```python
from build123d import *

# Parameters (mm, degrees)
ESBO_O1_W                = 23
ESBO_O1_H                = 23
RESSALTO_EXTRUS_O1_DEPTH = 10.25
CORTE_EXTRUS_O1_REACH    = 21.224
ESBO_O2_R                = 4.2
ESBO_O3_W                = 60
ESBO_O3_H                = 60
RESSALTO_EXTRUS_O2_DEPTH = 7
CORTE_EXTRUS_O2_REACH    = 45.647
ESBO_O4_R                = 1.5
CORTE_EXTRUS_O3_DEPTH    = 2.8
FILETE1_R                = 2
FILETE2_R                = 2


with BuildPart() as part:
    # Esboço1 → Ressalto-extrusão1 (new body)
    with BuildSketch(Plane.XY):
        Rectangle(ESBO_O1_W, ESBO_O1_H)
    extrude(amount=RESSALTO_EXTRUS_O1_DEPTH)

    # Esboço2 → Corte-extrusão1 (cut, up to next)
    with BuildSketch(Plane(origin=(0, 0, 0), x_dir=(-1, 0, 0), z_dir=(0, 0, -1)), mode=Mode.PRIVATE) as corte_extrus_o1_sk1:
        Circle(ESBO_O2_R)
    corte_extrus_o1_tool1 = extrude(corte_extrus_o1_sk1.sketch, amount=-CORTE_EXTRUS_O1_REACH, mode=Mode.PRIVATE) & part.part
    add(corte_extrus_o1_tool1.solids().sort_by_distance((0, 0, 0))[0], mode=Mode.SUBTRACT)

    # Esboço3 → Ressalto-extrusão2 (add)
    with BuildSketch(Plane.XY.offset(10.25)):
        Rectangle(ESBO_O3_W, ESBO_O3_H)
    extrude(amount=RESSALTO_EXTRUS_O2_DEPTH)

    # Esboço4 → Corte-extrusão2 (cut, up to next)
    with BuildSketch(Plane(origin=(0, 0, 10.25), x_dir=(-1, 0, 0), z_dir=(0, 0, -1)), mode=Mode.PRIVATE) as corte_extrus_o2_sk1:
        Circle(ESBO_O4_R)
    corte_extrus_o2_tool1 = extrude(corte_extrus_o2_sk1.sketch, amount=-CORTE_EXTRUS_O2_REACH, mode=Mode.PRIVATE) & part.part
    add(corte_extrus_o2_tool1.solids().sort_by_distance((0, 0, 10.25))[0], mode=Mode.SUBTRACT)

    # Esboço5 → Corte-extrusão3 (cut)
    with BuildSketch(Plane.XY.offset(17.25)):
        Polygon((3.290896534, 0), (1.645448267, 2.85), (-1.645448267, 2.85), (-3.290896534, 0), (-1.645448267, -2.85), (1.645448267, -2.85), align=None)
    extrude(amount=-CORTE_EXTRUS_O3_DEPTH, mode=Mode.SUBTRACT)

    # Filete1
    filete1_edges = [part.edges().sort_by_distance(p)[0] for p in [
        (-30, 0, 10.25),
        (0, -30, 10.25),
        (30, 0, 10.25),
        (0, 30, 10.25),
    ]]
    fillet(filete1_edges, radius=FILETE1_R)

    # Filete2
    # the kernel refuses this fillet: 2 mm, written as the material it takes off along each edge
    with BuildSketch(Plane(origin=(-28, -28, 12.25), x_dir=(-1, 0, 0), z_dir=(0, -1, 0))) as filete2_piece_1_section:
        Polygon((0, 0), (FILETE2_R, 0), (FILETE2_R, FILETE2_R), (0, FILETE2_R), align=None)
    filete2_piece_1 = extrude(amount=FILETE2_R, mode=Mode.PRIVATE)
    filete2_piece_1 = filete2_piece_1 - Plane(origin=(-28, -28, 12.25), x_dir=(0.7071067811865475, 0, 0.7071067811865475), z_dir=(0, -1, 0)) * Sphere(FILETE2_R, mode=Mode.PRIVATE)
    add(filete2_piece_1, mode=Mode.SUBTRACT)
    with BuildSketch(Plane(origin=(-28, 28, 12.25), x_dir=(0, 1, 0), z_dir=(-1, 0, 0))) as filete2_piece_2_section:
        Polygon((0, 0), (FILETE2_R, 0), (FILETE2_R, FILETE2_R), (0, FILETE2_R), align=None)
    filete2_piece_2 = extrude(amount=FILETE2_R, mode=Mode.PRIVATE)
    filete2_piece_2 = filete2_piece_2 - Plane(origin=(-28, 28, 12.25), x_dir=(0, -0.7071067811865475, 0.7071067811865475), z_dir=(-1, 0, 0)) * Sphere(FILETE2_R, mode=Mode.PRIVATE)
    add(filete2_piece_2, mode=Mode.SUBTRACT)
    with BuildSketch(Plane(origin=(28, -28, 12.25), x_dir=(1, 0, 0), z_dir=(0, -1, 0))) as filete2_piece_3_section:
        Polygon((0, 0), (FILETE2_R, 0), (FILETE2_R, -FILETE2_R), (0, -FILETE2_R), align=None)
    filete2_piece_3 = extrude(amount=FILETE2_R, mode=Mode.PRIVATE)
    filete2_piece_3 = filete2_piece_3 - Plane(origin=(28, -28, 12.25), x_dir=(-0.7071067811865475, 0, 0.7071067811865475), z_dir=(0, -1, 0)) * Sphere(FILETE2_R, mode=Mode.PRIVATE)
    add(filete2_piece_3, mode=Mode.SUBTRACT)
    with BuildSketch(Plane(origin=(28, 28, 12.25), x_dir=(0, 1, 0), z_dir=(1, 0, 0))) as filete2_piece_4_section:
        Polygon((0, 0), (FILETE2_R, 0), (FILETE2_R, -FILETE2_R), (0, -FILETE2_R), align=None)
    filete2_piece_4 = extrude(amount=FILETE2_R, mode=Mode.PRIVATE)
    filete2_piece_4 = filete2_piece_4 - Plane(origin=(28, 28, 12.25), x_dir=(0, -0.7071067811865475, 0.7071067811865475), z_dir=(1, 0, 0)) * Sphere(FILETE2_R, mode=Mode.PRIVATE)
    add(filete2_piece_4, mode=Mode.SUBTRACT)
    with BuildSketch(Plane(origin=(-30, 30, 12.25), x_dir=(0, -1, 0), z_dir=(0, 0, 1)), Plane(origin=(-30, -30, 12.25), x_dir=(1, 0, 0), z_dir=(0, 0, 1))) as filete2_piece_5:
        with BuildLine():
            CenterArc((FILETE2_R, FILETE2_R), FILETE2_R, 180, 90)
            Line((0, FILETE2_R), (0, 0))
            Line((0, 0), (FILETE2_R, 0))
        make_face()
    extrude(amount=10, mode=Mode.SUBTRACT)
    with BuildSketch(Plane(origin=(30, -30, 12.25), x_dir=(-1, 0, 0), z_dir=(0, 0, 1)), Plane(origin=(30, 30, 12.25), x_dir=(0, -1, 0), z_dir=(0, 0, 1))) as filete2_piece_6:
        with BuildLine():
            CenterArc((FILETE2_R, -FILETE2_R), FILETE2_R, 90, 90)
            Line((0, -FILETE2_R), (0, 0))
            Line((0, 0), (FILETE2_R, 0))
        make_face()
    extrude(amount=10, mode=Mode.SUBTRACT)


solid = part.part
```
For this review, take the finished solid that the model builds, in its own axes (mm). A direction names the side the tool comes from. Round coordinates to 2 decimals unless told otherwise and drop trailing zeros. Write each loop counter-clockwise with the first axis right and the second up, starting at its lowest first coordinate (ties: lowest second). Pieces come first, ordered by that corner, then holes. Notation, with made-up numbers: (1, 1) - (23, 1) arc R12 ccw to (23, 19) - close; hole circle Ø3 at (81, 75). An arc over 180 degrees is marked (long way). Answer as CSV lines item,"result". Start each with the question number.
(1) Add section A-A, the plane x = 0. State the section outline as (y, z) points.
(2) Mouldability with a two-part tool opening along X and no side actions: class faces 1 (the flat face through (0, -30, 15)), 2 (the flat face through (-30, 0, 15)), 3 (the flat face through (-2, 0, 14.45)), 4 (the flat face through (11.5, 0, 5)) as +X half, -X half, draft (parallel to the pull), parting line (faces both ways), or undercut.
(3) For pin 1 (5 mm diameter, centred on x = -22, y = 13, fed in from -Z); pin 2 (6 mm diameter, centred on y = 19, z = 7.5, fed in from +X); pin 3 (1 mm diameter, centred on y = -7.5, z = 3, fed in from -X), all flat-tipped, find the tip position at first contact; note any pin that passes through.
(4) For line 1 (Y direction, x = 0, z = 2.75); line 2 (Z direction, x = -1, y = 14.5); line 3 (X direction, y = -7.5, z = 2.25), list the stretches that pass through material, from the lowest coordinate up.
(5) Add section C-C, the plane z = 11.25. State the section outline as (x, y) points, plus the area to 3 significant figures.
(6) Add section B-B, the plane y = 6. State the section outline as (x, z) points.
(7) Machinability: for faces 5 (the cylindrical face through (-4.006, 1.262, 5.053)), 6 (the flat face through (0, 11.5, 5)), 7 (the flat face through (2.46, -1.44, 15.87)), which of the approach directions +Z, -Z, +X, -X, +Y, -Y give a long, thin tool a straight path to every point of the face, cutting with its end or side? Answer none if there is none.
From the geometry:
1,outline,"(-30, 12.25) arc R2 ccw to (-28, 10.25) - (-11.5, 10.25) - (-11.5, 0) - (-4.2, 0) - (-4.2, 10.25) - (-1.5, 10.25) - (-1.5, 14.45) - (-2.85, 14.45) - (-2.85, 17.25) - (-30, 17.25) - close; (1.5, 10.25) - (4.2, 10.25) - (4.2, 0) - (11.5, 0) - (11.5, 10.25) - (28, 10.25) arc R2 ccw to (30, 12.25) - (30, 17.25) - (2.85, 17.25) - (2.85, 14.45) - (1.5, 14.45) - close"
2,face 1,"draft"
2,face 2,"-X half"
2,face 3,"undercut"
2,face 4,"+X half"
3,pin 1,"stops at z = 10.25"
3,pin 2,"stops at x = 28.97"
3,pin 3,"stops at x = -11.5"
4,line 1,"y = -11.5 to -4.2, 4.2 to 11.5"
4,line 2,"z = 10.25 to 17.25"
4,line 3,"x = -11.5 to 11.5"
5,outline,"(-29.73, -28) arc R1.73 ccw to (-28, -29.73) - (28, -29.73) arc R1.73 ccw to (29.73, -28) - (29.73, 28) arc R1.73 ccw to (28, 29.73) - (-28, 29.73) arc R1.73 ccw to (-29.73, 28) - close; hole circle Ø3 at (0, 0)"
5,area,"3,530 mm²"
6,outline,"(-30, 12.25) arc R2 ccw to (-28, 10.25) - (-11.5, 10.25) - (-11.5, 0) - (11.5, 0) - (11.5, 10.25) - (28, 10.25) arc R2 ccw to (30, 12.25) - (30, 17.25) - (-30, 17.25) - close"
7,face 5,"-Z"
7,face 6,"-Z, +X, -X, +Y"
7,face 7,"+Z"
